The listing builds one solid part. Answer for the finished solid, in the listing's coordinates (mm). Face numbers are marked on the shaded views. A direction names the side the tool comes from. Give positions to 0.01 mm unless a question says otherwise; leave off trailing zeros. Order: outer loops, then holes, each group sorted by start corner. A loop starts at its lowest first (then second) coordinate and runs counter-clockwise, first axis right, second up. Notation, with made-up numbers: (57.5, -12) - (105.5, -12) arc R11 cw to (105.5, 1) - close; hole circle Ø8 at (62, 55). An arc over 180 degrees is marked (long way). Use CSV: the item, a comma, the result in double quotes.
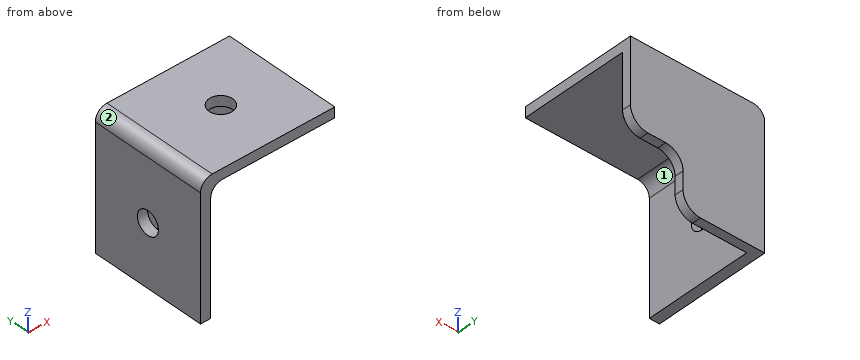
```python
from build123d import *

# Parameters (mm, degrees)
SALIENTE_EXTRUIR1_DEPTH = 20
CORTAR_EXTRUIR1_DEPTH   = 18.5
REDONDEO1_R             = 2
REDONDEO2_R             = 3
CROQUIS3_R              = 2
CORTAR_EXTRUIR2_DEPTH   = 18.5
CROQUIS4_R              = 2
CORTAR_EXTRUIR3_DEPTH   = 18.5


with BuildPart() as part:
    # Croquis1 → Saliente-Extruir1 (new body)
    with BuildSketch(Plane(origin=(0, 0, 0), x_dir=(1, 0, 0), z_dir=(0, 1, 0))):
        Polygon((0, 0), (23, 0), (23, 14), (14, 14), (14, 23), (0, 23), align=None)
    extrude(amount=SALIENTE_EXTRUIR1_DEPTH)

    # Croquis2 → Cortar-Extruir1 (cut)
    with BuildSketch(Plane.XZ):
        Polygon((1.75, -23), (1.75, -1.75), (23, -1.75), (23, -14), (14, -14), (14, -23), align=None)
    extrude(amount=-CORTAR_EXTRUIR1_DEPTH, mode=Mode.SUBTRACT)

    # Redondeo1
    redondeo1_edges = [part.edges().sort_by_distance(p)[0] for p in [
        (0, 10, 0),
        (1.75, 9.25, -1.75),
    ]]
    fillet(redondeo1_edges, radius=REDONDEO1_R)

    # Redondeo2
    redondeo2_edges = [part.edges().sort_by_distance(p)[0] for p in [
        (14, 19.25, -23),
        (14, 19.25, -14),
        (23, 19.25, -14),
    ]]
    fillet(redondeo2_edges, radius=REDONDEO2_R)

    # Croquis3 → Cortar-Extruir2 (cut)
    with BuildSketch(Plane.ZY):
        with Locations((-12.5, 10)):
            Circle(CROQUIS3_R)
    extrude(amount=-CORTAR_EXTRUIR2_DEPTH, mode=Mode.SUBTRACT)

    # Croquis4 → Cortar-Extruir3 (cut)
    with BuildSketch(Plane.XY):
        with Locations((12.5, 10)):
            Circle(CROQUIS4_R)
    extrude(amount=-CORTAR_EXTRUIR3_DEPTH, mode=Mode.SUBTRACT)


solid = part.part
```
Item 1: The part is cut by section D-D (y = 2). Give the vertices of the cut face in (x, z), and give its area (3 significant figures).
Taken from the geometry:
outline,"(0, -23) - (1.75, -23) - (1.75, -3.75) arc R2 cw to (3.75, -1.75) - (23, -1.75) - (23, 0) - (2, 0) arc R2 ccw to (0, -2) - close"
area,"77.4 mm^2"
Item 2: The part is cut by section B-B (z = -12.5). Give the vertices of the cut face in (x, y).
Taken from the geometry:
outline,"(0, 0) - (1.75, 0) - (1.75, 8) - (0, 8) - close; (0, 12) - (1.75, 12) - (1.75, 18.5) - (22.6, 18.5) - (22.6, 20) - (0, 20) - close"
Item 3: The part is cut by section A-A (y = 10). Give the vertices of the cut face in (x, z).
Taken from the geometry:
outline,"(0, -23) - (1.75, -23) - (1.75, -14.5) - (0, -14.5) - close; (0, -10.5) - (1.75, -10.5) - (1.75, -3.75) arc R2 cw to (3.75, -1.75) - (10.5, -1.75) - (10.5, 0) - (2, 0) arc R2 ccw to (0, -2) - close; (14.5, -1.75) - (23, -1.75) - (23, 0) - (14.5, 0) - close"
Item 4: Which of the six approach directions +Z, -Z, +X, -X, +Y, -Y give full straight-line access (tool end or side, diameter ignored) to the marked faces 1 and 2?
Taken from the geometry:
face 1,"-Z, +X, -Y"
face 2,"+Z, -X, +Y, -Y"
Item 5: Each of these flat-tipped pins is pushed along its axis until it touches: pin 1 (2 mm diameter, centred on y = 4, z = -15, fed in from +X); pin 2 (1.5 mm diameter, centred on x = 20, y = 5.5, fed in from -Z); pin 3 (0.8 mm diameter, centred on y = 19, z = -19, fed in from +X). Where does it stop, or does it pass through?
Taken from the geometry:
pin 1,"x = 1.75"
pin 2,"z = -1.75"
pin 3,"x = 14"
Item 6: The part is cut by section C-C (x = 4.75). Give the vertices of the cut face in (y, z), and give its area (3 significant figures).
Taken from the geometry:
outline,"(0, -1.75) - (18.5, -1.75) - (18.5, -23) - (20, -23) - (20, 0) - (0, 0) - close"
area,"66.9 mm^2"
Item 7: Find the intervals of material crossed by line 1 along Y through (x, z) = (12.5, -1); line 2 along Z through (x, y) = (21.75, 16.5); line 3 along X through (y, z) = (16.5, -21.75), in increasing order.
Taken from the geometry:
line 1,"0 to 8, 12 to 20"
line 2,"-1.75 to 0"
line 3,"0 to 1.75"
